Source: CAD feature listing. Evaluate the final solid. Frame: model axes, mm. Give positions to 0.01 mm unless a question says otherwise; leave off trailing zeros. Order: outer loops, then holes, each group sorted by start corner. A loop starts at its lowest first (then second) coordinate and runs counter-clockwise, first axis right, second up. Notation, with made-up numbers: M 57.25,-1 L 115.25,-1 A12 cw 115.25,16 Z; hole C 87,-16 d4. An arc over 180 degrees is marked long. Use CSV: the item, a comma, the result in double quotes. Start each with the question number.
1. Line query: line 1 along Y through (x, z) = (38.5, 0.8); line 2 along X through (y, z) = (20, 1.2). Output: solid intervals per line, ascending. Write a range as [from, to].
2. Section query B-B, the plane x = 38. Return the cut outline in (y, z).
3. Section query C-C, the plane z = 0.4. State how many separate pieces and enclosed holes the cut face has, plus the area to 4 significant figures.
4. Pin query (flat end, axial travel): P1, Ø4, axis at x = -37.5, y = 8.5, coming from the +Z side. Return the tip coordinate at first contact, or that it passes through.
5. Section query A-A, the plane y = 8.5. Return the cut outline in (x, z), plus the area to 3 significant figures.
Solid Edge part; units mm, degrees
sketch "Sketch1" plane through (0, 0, 0) normal (0, 0, 1) x (1, 0, 0)
  line L0 (-48, 45) -> (-48, -45)
  line L1 (-48, -45) -> (48, -45)
  line L2 (48, -45) -> (48, 45)
  line L3 (48, 45) -> (-48, 45)
extrude "Protrusion1" add sketch "Sketch1" along normal blind 1.5
sketch "Sketch2" plane through (0, 0, 0) normal (0, 0, -1) x (1, 0, 0)
  line L0 (-31.5, 17.5) -> (-31.5, 40.5)
  line L1 (-31.5, 40.5) -> (-44.5, 40.5)
  line L2 (-44.5, 40.5) -> (-44.5, 17.5)
  line L3 (-44.5, 17.5) -> (-31.5, 17.5)
  line L4 (-25.5, 17.5) -> (-12.5, 17.5)
  line L5 (-12.5, 17.5) -> (-12.5, 40.5)
  line L6 (-12.5, 40.5) -> (-25.5, 40.5)
  line L7 (-25.5, 40.5) -> (-25.5, 17.5)
  line L8 (-6.5, 17.5) -> (6.5, 17.5)
  line L9 (6.5, 17.5) -> (6.5, 40.5)
  line L10 (6.5, 40.5) -> (-6.5, 40.5)
  line L11 (-6.5, 40.5) -> (-6.5, 17.5)
  line L12 (12.5, 17.5) -> (25.5, 17.5)
  line L13 (25.5, 17.5) -> (25.5, 40.5)
  line L14 (25.5, 40.5) -> (12.5, 40.5)
  line L15 (12.5, 40.5) -> (12.5, 17.5)
  line L16 (31.5, 17.5) -> (44.5, 17.5)
  line L17 (44.5, 17.5) -> (44.5, 40.5)
  line L18 (44.5, 40.5) -> (31.5, 40.5)
  line L19 (31.5, 40.5) -> (31.5, 17.5)
  line L20 (44.5, 11.5) -> (31.5, 11.5)
  line L21 (31.5, 11.5) -> (31.5, -11.5)
  line L22 (31.5, -11.5) -> (44.5, -11.5)
  line L23 (44.5, -11.5) -> (44.5, 11.5)
  line L24 (25.5, 11.5) -> (12.5, 11.5)
  line L25 (12.5, 11.5) -> (12.5, -11.5)
  line L26 (12.5, -11.5) -> (25.5, -11.5)
  line L27 (25.5, -11.5) -> (25.5, 11.5)
  line L28 (6.5, 11.5) -> (-6.5, 11.5)
  line L29 (-6.5, 11.5) -> (-6.5, -11.5)
  line L30 (-6.5, -11.5) -> (6.5, -11.5)
  line L31 (6.5, -11.5) -> (6.5, 11.5)
  line L32 (-12.5, 11.5) -> (-25.5, 11.5)
  line L33 (-25.5, 11.5) -> (-25.5, -11.5)
  line L34 (-25.5, -11.5) -> (-12.5, -11.5)
  line L35 (-12.5, -11.5) -> (-12.5, 11.5)
  line L36 (-31.5, 11.5) -> (-44.5, 11.5)
  line L37 (-44.5, 11.5) -> (-44.5, -11.5)
  line L38 (-44.5, -11.5) -> (-31.5, -11.5)
  line L39 (-31.5, -11.5) -> (-31.5, 11.5)
  line L40 (-44.5, -17.5) -> (-44.5, -40.5)
  line L41 (-44.5, -40.5) -> (-31.5, -40.5)
  line L42 (-31.5, -40.5) -> (-31.5, -17.5)
  line L43 (-31.5, -17.5) -> (-44.5, -17.5)
  line L44 (-12.5, -17.5) -> (-25.5, -17.5)
  line L45 (-25.5, -17.5) -> (-25.5, -40.5)
  line L46 (-25.5, -40.5) -> (-12.5, -40.5)
  line L47 (-12.5, -40.5) -> (-12.5, -17.5)
  line L48 (-6.5, -17.5) -> (-6.5, -40.5)
  line L49 (-6.5, -40.5) -> (6.5, -40.5)
  line L50 (6.5, -40.5) -> (6.5, -17.5)
  line L51 (6.5, -17.5) -> (-6.5, -17.5)
  line L52 (12.5, -17.5) -> (12.5, -40.5)
  line L53 (12.5, -40.5) -> (25.5, -40.5)
  line L54 (25.5, -40.5) -> (25.5, -17.5)
  line L55 (25.5, -17.5) -> (12.5, -17.5)
  line L56 (31.5, -17.5) -> (31.5, -40.5)
  line L57 (31.5, -40.5) -> (44.5, -40.5)
  line L58 (44.5, -40.5) -> (44.5, -17.5)
  line L59 (44.5, -17.5) -> (31.5, -17.5)
extrude "ExtrudedCutout_1" cut sketch "Sketch2" along normal mid plane 80
Result set:
1,line 1,"[-45, -40.5], [-17.5, -11.5], [11.5, 17.5], [40.5, 45]"
1,line 2,"[-48, -44.5], [-31.5, -25.5], [-12.5, -6.5], [6.5, 12.5], [25.5, 31.5], [44.5, 48]"
2,outline,"M -45,0 L -40.5,0 L -40.5,1.5 L -45,1.5 Z; M -17.5,0 L -11.5,0 L -11.5,1.5 L -17.5,1.5 Z; M 11.5,0 L 17.5,0 L 17.5,1.5 L 11.5,1.5 Z; M 40.5,0 L 45,0 L 45,1.5 L 40.5,1.5 Z"
3,separate pieces,"1"
3,enclosed holes,"15"
3,area,"4,155 mm2"
4,P1,"through"
5,outline,"M -48,0 L -44.5,0 L -44.5,1.5 L -48,1.5 Z; M -31.5,0 L -25.5,0 L -25.5,1.5 L -31.5,1.5 Z; M -12.5,0 L -6.5,0 L -6.5,1.5 L -12.5,1.5 Z; M 6.5,0 L 12.5,0 L 12.5,1.5 L 6.5,1.5 Z; M 25.5,0 L 31.5,0 L 31.5,1.5 L 25.5,1.5 Z; M 44.5,0 L 48,0 L 48,1.5 L 44.5,1.5 Z"
5,area,"46.5 mm2"
